Check sheet for the drawn part. Datum: minimum x, y, z corner. Units: mm. Give positions to 0.01 mm unless a question says otherwise; leave off trailing zeros. Loops run counter-clockwise (first coordinate to the right, second up) from the corner with the lowest first, then second, coordinate; pieces in that order, holes last. Notation, with made-up numbers: (1.5, -39) - (9.5, -39) arc R23 ccw to (9.5, -1) - close; hole circle Ø5 at (-16, 75). An arc over 180 degrees is marked (long way). One line per item, written item: value. Start each with the question number.
1. Sectioned sample at B-B (z = 3). Record the cut outline in (x, y).
2. Sectioned sample at D-D (x = 199). Record the cut outline in (y, z).
3. Scan lines: L1, parallel to Y at x = 156.5, z = 1.8; L2, parallel to Y at x = 156.5, z = 8.2; L3, parallel to X at y = 96.5, z = 2.4. Record each from-to range of solid material in increasing order. Write a range as [from, to].
4. Sectioned sample at A-A (y = 181.5). Record the cut outline in (x, z), plus the area to 4 significant figures.
5. Gauge pin test, flat ends, axial feed: pin 1 (7 mm diameter, centred on x = 156.5, y = 96.5, fed in from +Z); pin 2 (5.5 mm diameter, centred on y = 113.5, z = 1.5, fed in from +X); pin 3 (6 mm diameter, centred on x = 137.5, y = 213, fed in from -Z); pin 4 (2.5 mm diameter, centred on x = 156, y = 183, fed in from +Z). Record the tip position at first contact, or that the pin passes through.
6. Sectioned sample at C-C (x = 81.5). Record the cut outline in (y, z), plus the area to 4 significant figures.
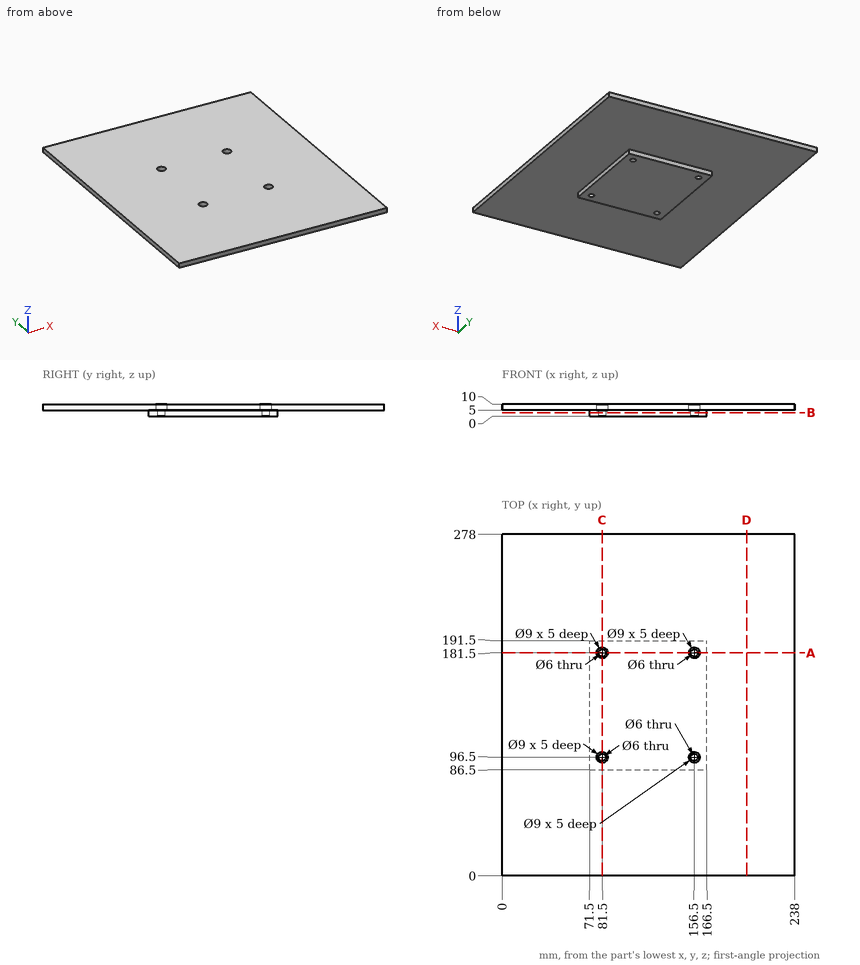
Results are:
1. outline: (71.5, 86.5) - (166.5, 86.5) - (166.5, 191.5) - (71.5, 191.5) - close; hole circle Ø6 at (81.5, 96.5); hole circle Ø6 at (81.5, 181.5); hole circle Ø6 at (156.5, 96.5); hole circle Ø6 at (156.5, 181.5)
2. outline: (0, 5) - (278, 5) - (278, 10) - (0, 10) - close
3. L1: y = [86.5, 93.5], [99.5, 178.5], [184.5, 191.5]
3. L2: y = [0, 92], [101, 177], [186, 278]
3. L3: x = [71.5, 78.5], [84.5, 153.5], [159.5, 166.5]
4. outline: (0, 5) - (71.5, 5) - (71.5, 0) - (78.5, 0) - (78.5, 5) - (77, 5) - (77, 10) - (0, 10) - close; (84.5, 0) - (153.5, 0) - (153.5, 5) - (152, 5) - (152, 10) - (86, 10) - (86, 5) - (84.5, 5) - close; (159.5, 0) - (166.5, 0) - (166.5, 5) - (238, 5) - (238, 10) - (161, 10) - (161, 5) - (159.5, 5) - close
4. area: 1,515 mm^2
5. pin 1: stops at z = 5
5. pin 2: stops at x = 166.5
5. pin 3: stops at z = 5
5. pin 4: passes through
6. outline: (0, 5) - (86.5, 5) - (86.5, 0) - (93.5, 0) - (93.5, 5) - (92, 5) - (92, 10) - (0, 10) - close; (99.5, 0) - (178.5, 0) - (178.5, 5) - (177, 5) - (177, 10) - (101, 10) - (101, 5) - (99.5, 5) - close; (184.5, 0) - (191.5, 0) - (191.5, 5) - (278, 5) - (278, 10) - (186, 10) - (186, 5) - (184.5, 5) - close
6. area: 1,765 mm^2
